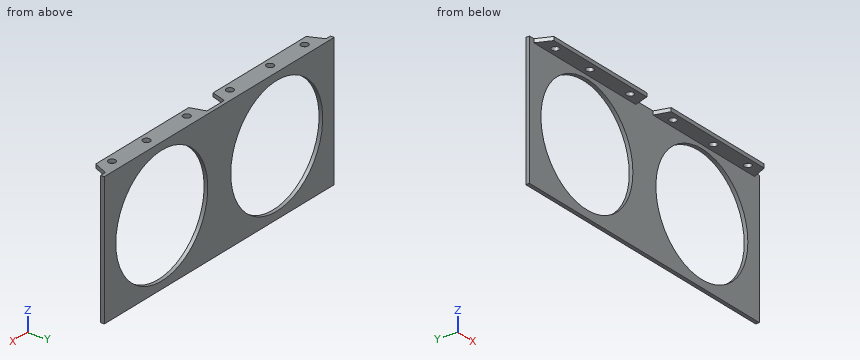
```python
from build123d import *

# Parameters (mm, degrees)
F0_W     = 254
F0_H     = 114.3
F0_R     = 50.8
F1_DEPTH = 3.175
F2_W     = 112.5140171498
F2_H     = 3.175
F2_W_2   = 112.2281569988
F3_DEPTH = 12.7
F5_DEPTH = 25.4
F7_DEPTH = 25.4


with BuildPart() as f1:
    # F0 (on Front) → F1 (new body)
    with BuildSketch(Plane.XZ):
        Rectangle(F0_W, F0_H)
        with Locations((-63.5, 0)):
            Circle(F0_R, mode=Mode.SUBTRACT)
        with Locations((63.5, 0)):
            Circle(F0_R, mode=Mode.SUBTRACT)
    extrude(amount=F1_DEPTH)

    # F2 (on face) → F3 (join)
    with BuildSketch(Plane.XZ.offset(3.175)):
        with Locations((-65.7536098734, 55.5625)):
            Rectangle(F2_W, F2_H)
        with Locations((65.7025436531, 55.5625)):
            Rectangle(F2_W_2, F2_H)
    extrude(amount=F3_DEPTH)

    # F4 (on face) → F5 (cut)
    with BuildSketch(Plane.XY.offset(57.15)):
        Polygon((-116.2076666951, -15.875), (-122.0106184483, -3.175), (-122.0106184483, -15.875), align=None)
        Polygon((-9.4966012985, -15.875), (-9.4966012985, -3.175), (-13.4629756212, -15.875), align=None)
        Polygon((13.4817082435, -15.875), (9.5884651538, -3.175), (9.5884651538, -15.875), align=None)
        Polygon((116.2402704358, -15.875), (121.8166221525, -15.875), (121.8166221525, -3.175), align=None)
    extrude(amount=-F5_DEPTH, mode=Mode.SUBTRACT)

    # F6 (on face) → F7 (cut)
    with BuildSketch(Plane.XY.offset(57.15)):
        with BuildLine():
            ThreePointArc((-103.2341425717, -9.525), (-106.4091425717, -6.35), (-109.5841425717, -9.525))
            Line((-109.5841425717, -9.525), (-103.2341425717, -9.525))
        make_face()
        with BuildLine():
            ThreePointArc((109.5034462942, -9.525), (106.3284462942, -6.35), (103.1534462942, -9.525))
            Line((103.1534462942, -9.525), (109.5034462942, -9.525))
        make_face()
        with BuildLine():
            Line((109.5034462942, -9.525), (103.1534462942, -9.525))
            ThreePointArc((103.1534462942, -9.525), (106.3284462942, -12.7), (109.5034462942, -9.525))
        make_face()
        with BuildLine():
            ThreePointArc((71.4034462942, -9.525), (68.2284462942, -6.35), (65.0534462942, -9.525))
            Line((65.0534462942, -9.525), (71.4034462942, -9.525))
        make_face()
        with BuildLine():
            Line((71.4034462942, -9.525), (65.0534462942, -9.525))
            ThreePointArc((65.0534462942, -9.525), (68.2284462942, -12.7), (71.4034462942, -9.525))
        make_face()
        with BuildLine():
            ThreePointArc((26.9534462942, -9.525), (23.7784462942, -6.35), (20.6034462942, -9.525))
            Line((20.6034462942, -9.525), (26.9534462942, -9.525))
        make_face()
        with BuildLine():
            Line((26.9534462942, -9.525), (20.6034462942, -9.525))
            ThreePointArc((20.6034462942, -9.525), (23.7784462942, -12.7), (26.9534462942, -9.525))
        make_face()
        with BuildLine():
            ThreePointArc((-20.6841425717, -9.525), (-23.8591425717, -6.35), (-27.0341425717, -9.525))
            Line((-27.0341425717, -9.525), (-20.6841425717, -9.525))
        make_face()
        with BuildLine():
            Line((-20.6841425717, -9.525), (-27.0341425717, -9.525))
            ThreePointArc((-27.0341425717, -9.525), (-23.8591425717, -12.7), (-20.6841425717, -9.525))
        make_face()
        with BuildLine():
            ThreePointArc((-65.1341425717, -9.525), (-68.3091425717, -6.35), (-71.4841425717, -9.525))
            Line((-71.4841425717, -9.525), (-65.1341425717, -9.525))
        make_face()
        with BuildLine():
            Line((-65.1341425717, -9.525), (-71.4841425717, -9.525))
            ThreePointArc((-71.4841425717, -9.525), (-68.3091425717, -12.7), (-65.1341425717, -9.525))
        make_face()
        with BuildLine():
            Line((-103.2341425717, -9.525), (-109.5841425717, -9.525))
            ThreePointArc((-109.5841425717, -9.525), (-106.4091425717, -12.7), (-103.2341425717, -9.525))
        make_face()
    extrude(amount=-F7_DEPTH, mode=Mode.SUBTRACT)


solid = f1.part
```
Work out the finished part from the listing and answer in its coordinate system (mm). Give positions to 0.01 mm unless a question says otherwise; leave off trailing zeros. Order: outer loops, then holes, each group sorted by start corner. A loop starts at its lowest first (then second) coordinate and runs counter-clockwise, first axis right, second up.
1. Section A-A, the plane z = 0 is taken. Determine the outline of the cut face in (x, y) (3 decimals), and give its area (3 significant figures).
Result sheet:
outline: (-127, -3.175) - (-114.3, -3.175) - (-114.3, 0) - (-127, 0) - close; (-12.7, -3.175) - (12.7, -3.175) - (12.7, 0) - (-12.7, 0) - close; (114.3, -3.175) - (127, -3.175) - (127, 0) - (114.3, 0) - close
area: 161 mm2
2. Section C-C, the plane z = -18 is taken. Determine the outline of the cut face in (x, y) (3 decimals).
Result sheet:
outline: (-127, -3.175) - (-111.004, -3.175) - (-111.004, 0) - (-127, 0) - close; (-15.996, -3.175) - (15.996, -3.175) - (15.996, 0) - (-15.996, 0) - close; (111.004, -3.175) - (127, -3.175) - (127, 0) - (111.004, 0) - close
3. Straight lines are drawn through the part: L1, parallel to X at y = -2.25, z = 3; L2, parallel to X at y = -3, z = -20.5; L3, parallel to Z at x = 70, y = -3.75 (3 decimals). For each, find the intervals that lie inside material, in ascending order.
Result sheet:
L1: x = -127 to -114.21, -12.79 to 12.79, 114.21 to 127
L2: x = -127 to -109.98, -17.02 to 17.02, 109.98 to 127
L3: z = 53.975 to 57.15
4. Section B-B, the plane x = -106.5 is taken. Determine the outline of the cut face in (y, z) (3 decimals), and give its area (3 significant figures).
Result sheet:
outline: (-15.875, 53.975) - (-12.699, 53.975) - (-12.699, 57.15) - (-15.875, 57.15) - close; (-6.351, 53.975) - (-3.175, 53.975) - (-3.175, 27.049) - (0, 27.049) - (0, 57.15) - (-6.351, 57.15) - close; (-3.175, -57.15) - (0, -57.15) - (0, -27.049) - (-3.175, -27.049) - close
area: 211 mm2
5. Each of these flat-tipped pins is pushed along its axis until it touches: P1, Ø8.5, axis at x = -23.86, y = -9.52, coming from the -Z side (3 decimals); P2, Ø8, axis at x = 57.5, z = -44, coming from the +Y side; P3, Ø10, axis at x = 4.5, z = -38.5, coming from the +Y side. Where does it stop, or does it pass through?
Result sheet:
P1: stops at z = 53.975
P2: passes through
P3: stops at y = 0
